```python
from build123d import *
from OCP.BRepFilletAPI import BRepFilletAPI_MakeChamfer

# Parameters (mm, degrees)
BOSS_EXTRU_1_DEPTH           = 5
ESQUISSE2_R                  = 5.1
ESQUISSE2_R_2                = 2.1
ENL_V_MAT_EXTRU_1_DEPTH      = 91.691785736
ESQUISSE3_W                  = 32
ESQUISSE3_H                  = 20
BOSS_EXTRU_2_DEPTH           = 26
CHANFREIN1_SIZE              = 10
CHANFREIN1_SIZE_2            = 26
CONG_1_R                     = 10
ESQUISSE4_W                  = 18
ESQUISSE4_H                  = 20
ENL_V_MAT_EXTRU_2_DEPTH      = 26
CONG_2_R                     = 2
ENL_V_MAT_EXTRU_3_DEPTH      = 105.220919205
ENL_V_MAT_EXTRU_3_DEPTH_BACK = 105.220919205
ESQUISSE5_R                  = 2.1
ENL_V_START                  = -8
ESQUISSE6_R                  = 8
ENL_V_MAT_EXTRU_4_DEPTH      = 26
ESQUISSE7_R                  = 8
ENL_V_MAT_EXTRU_5_DEPTH      = 97.220919205
CONG_3_START                 = -11
CONG_3_DEPTH                 = 22
SKETCH1_R                    = 2.1
CUT_EXTRUDE1_DEPTH           = 95.212525707


with BuildPart() as part:
    # Esquisse1 → Boss.-Extru.1 (new body)
    with BuildSketch(Plane.XY):
        with BuildLine():
            Line((-80, 10), (80, 10))
            ThreePointArc((80, 10), (90, 0), (80, -10))
            Line((80, -10), (-80, -10))
            ThreePointArc((-80, -10), (-90, 0), (-80, 10))
        make_face()
    extrude(amount=BOSS_EXTRU_1_DEPTH)

    # Esquisse2 → Enlèv. mat.-Extru.1 (cut, through all)
    with BuildSketch(Plane.XY.offset(5)):
        with Locations((-80, 0)):
            Circle(ESQUISSE2_R)
        with Locations((80, 0)):
            Circle(ESQUISSE2_R)
        with Locations((-50, 0)):
            Circle(ESQUISSE2_R_2)
        with Locations((50, 0)):
            Circle(ESQUISSE2_R_2)
    extrude(amount=-ENL_V_MAT_EXTRU_1_DEPTH, mode=Mode.SUBTRACT)

    # Esquisse3 → Boss.-Extru.2 (add)
    with BuildSketch(Plane.XY.offset(5)):
        Rectangle(ESQUISSE3_W, ESQUISSE3_H)
    extrude(amount=BOSS_EXTRU_2_DEPTH)

    # Chanfrein1
    chanfrein1_edges_1 = [part.edges().sort_by_distance(p)[0] for p in [
        (16, 0, 5),
    ]]
    chanfrein1_side_1 = [part.faces().sort_by_distance(p)[0] for p in [
        (16.2, 0, 5),
    ]]
    chanfrein1_edges_2 = [part.edges().sort_by_distance(p)[0] for p in [
        (-16, 0, 5),
    ]]
    chanfrein1_side_2 = [part.faces().sort_by_distance(p)[0] for p in [
        (-16.2, 0, 5),
    ]]
    chanfrein1 = BRepFilletAPI_MakeChamfer(part.part.solid().wrapped)
    for e in chanfrein1_edges_1:
        chanfrein1.Add(CHANFREIN1_SIZE - 0.0001, CHANFREIN1_SIZE_2 - 0.0001, e.wrapped, chanfrein1_side_1[0].wrapped)
    for e in chanfrein1_edges_2:
        chanfrein1.Add(CHANFREIN1_SIZE - 0.0001, CHANFREIN1_SIZE_2 - 0.0001, e.wrapped, chanfrein1_side_2[0].wrapped)
    add(Compound.cast(chanfrein1.Shape()), mode=Mode.REPLACE)  # a hair under: the kernel refuses the full size

    # Congé1
    cong_1_edges = [part.edges().sort_by_distance(p)[0] for p in [
        (25.9999, 0, 5),
        (-25.9999, 0, 5),
    ]]
    fillet(cong_1_edges, radius=CONG_1_R)

    # Esquisse4 → Enlèv. mat.-Extru.2 (cut)
    with BuildSketch(Plane.XY.offset(31)):
        Rectangle(ESQUISSE4_W, ESQUISSE4_H)
    extrude(amount=-ENL_V_MAT_EXTRU_2_DEPTH, mode=Mode.SUBTRACT)

    # Congé2
    cong_2_edges = [part.edges().sort_by_distance(p)[0] for p in [
        (9, 0, 5),
        (-9, 0, 5),
    ]]
    fillet(cong_2_edges, radius=CONG_2_R)

    # Esquisse5 → Enlèv. mat.-Extru.3 (cut, two sides: drawn at the far end of the back side and taken through both)
    with BuildSketch(Plane.ZY.offset(-9).offset(-ENL_V_MAT_EXTRU_3_DEPTH_BACK)):
        with Locations((24, 0)):
            Circle(ESQUISSE5_R)
    extrude(amount=ENL_V_MAT_EXTRU_3_DEPTH + ENL_V_MAT_EXTRU_3_DEPTH_BACK, mode=Mode.SUBTRACT)

    # Esquisse6 → Enlèv. mat.-Extru.4 (cut)
    with BuildSketch(Plane.ZY.offset(-9).offset(ENL_V_START)):
        with Locations((24, 0)):
            Circle(ESQUISSE6_R)
    extrude(amount=-ENL_V_MAT_EXTRU_4_DEPTH, mode=Mode.SUBTRACT)

    # Esquisse7 → Enlèv. mat.-Extru.5 (cut, through all)
    with BuildSketch(Plane(origin=(-9, 0, 0), x_dir=(0, 0, -1), z_dir=(1, 0, 0)).offset(ENL_V_START)):
        with Locations((-24, 0)):
            Circle(ESQUISSE7_R)
    extrude(amount=-ENL_V_MAT_EXTRU_5_DEPTH, mode=Mode.SUBTRACT)

    # Congé3: read off the stored shape, not the designer's step
    # Congé3 outline → Congé3 (cut)
    with BuildSketch(Plane(origin=(0, 0, 0), x_dir=(1, 0, 0), z_dir=(0, 1, 0)).offset(CONG_3_START)):
        with BuildLine():
            Line((-9, -31), (-9, -29))
            ThreePointArc((-9, -29), (-9.585786438, -30.414213562), (-11, -31))
            Line((-11, -31), (-9, -31))
        make_face()
        with BuildLine():
            Line((-16, -31), (-14.626401804, -31))
            ThreePointArc((-14.626401804, -31), (-15.758674669, -30.64862311), (-16.493093016, -29.717958159))
            Line((-16.493093016, -29.717958159), (-16, -31))
        make_face()
        with BuildLine():
            ThreePointArc((16.493093016, -29.717958159), (15.758674669, -30.64862311), (14.626401804, -31))
            Line((14.626401804, -31), (16, -31))
            Line((16, -31), (16.493093016, -29.717958159))
        make_face()
        with BuildLine():
            ThreePointArc((11, -31), (9.585786438, -30.414213562), (9, -29))
            Line((9, -29), (9, -31))
            Line((9, -31), (11, -31))
        make_face()
    extrude(amount=CONG_3_DEPTH, mode=Mode.SUBTRACT)

    # Sketch1 → Cut-Extrude1 (cut, through all)
    with BuildSketch(Plane.XY.offset(5)):
        Circle(SKETCH1_R)
    extrude(amount=-CUT_EXTRUDE1_DEPTH, mode=Mode.SUBTRACT)


solid = part.part
```
Check sheet for the modelled part. Datum: model origin and axes. Units: mm. A direction names the side the tool comes from. Round coordinates to 2 decimals unless told otherwise and drop trailing zeros. Order: outer loops, then holes, each group sorted by start corner. A loop starts at its lowest first (then second) coordinate and runs counter-clockwise, first axis right, second up.
1) Mould release check, pull along X, two halves, no side actions. Record for faces 5 (the flat face through (-17, -2, 22)), 6 (the flat face through (-0.1, 2.4, 5)), 7 (the cylindrical face through (-12.944, 0.631, 26.003)): +X half, -X half, draft (parallel to the pull), parting line (faces both ways), or undercut.
2) Section check C-C (y = 0). Give the number of separate pieces and of enclosed holes in the cut face, and give its area (3 significant figures).
3) Tool access check on faces 1 (the cylindrical face through (-19, 0, 16)), 2 (the flat face through (-9, 0, 18)), 3 (the flat face through (62, 0, 5)), 4 (the flat face through (17, -2, 22)). Record the directions out of +Z, -Z, +X, -X, +Y, -Y that give a thin tool (end or side, any length) a straight path to the whole face; none if there is none.
4) Section check D-D (z = 24). Record the boundary of the cut face in (x, y), and give its area (3 significant figures).
5) Section check B-B (z = 13.5). Record the boundary of the cut face in (x, y).
6) Scan lines: line 1 (X direction, y = 2.75, z = 19); line 2 (X direction, y = -3.5, z = 4); line 3 (Y direction, x = 0, z = 2.8). Record each from-to range of solid material in increasing order.
7) Go/stop test with flat-tipped pins: pin 1 Ø3.5 at (x, y) = (50, 0) entering from -Z; pin 2 Ø3 at (y, z) = (4.5, 11) entering from -X; pin 3 Ø8 at (y, z) = (-8, 10.5) entering from -X; pin 4 Ø4 at (x, y) = (40.5, -5) entering from +Z. Record where each tip stops, or that it passes through.
8) Section check A-A (x = 0). Record the boundary of the cut face in (y, z), and give its area (3 significant figures).
Result:
1. face 5: -X half
1. face 6: undercut
1. face 7: draft
2. separate pieces: 8
2. enclosed holes: 0
2. area: 1,250 mm2
3. face 1: -X
3. face 2: +Z, +Y, -Y
3. face 3: +Z, +X, +Y, -Y
3. face 4: +X
4. outline: (-18.69, -10) - (-9, -10) - (-9, -2.1) - (-17, -2.1) - (-17, -8) - (-18.69, -8) - close; (-18.69, 8) - (-17, 8) - (-17, 2.1) - (-9, 2.1) - (-9, 10) - (-18.69, 10) - close; (9, -10) - (18.69, -10) - (18.69, -8) - (17, -8) - (17, -2.1) - (9, -2.1) - close; (9, 2.1) - (17, 2.1) - (17, 8) - (18.69, 8) - (18.69, 10) - (9, 10) - close
4. area: 266 mm2
5. outline: (-22.73, -10) - (-9, -10) - (-9, 10) - (-22.73, 10) - close; (9, -10) - (22.73, -10) - (22.73, 10) - (9, 10) - close
6. line 1: x = -17 to -9, 9 to 17
6. line 2: x = -89.37 to -83.71, -76.29 to 76.29, 83.71 to 89.37
6. line 3: y = -10 to -2.1, 2.1 to 10
7. pin 1: passes through
7. pin 2: stops at x = -24.52
7. pin 3: stops at x = -27.6
7. pin 4: stops at z = 5
8. outline: (-10, 0) - (-2.1, 0) - (-2.1, 5) - (-10, 5) - close; (2.1, 0) - (10, 0) - (10, 5) - (2.1, 5) - close
8. area: 79.0 mm2
